Autodesk Inventor part; units mm, degrees
ref_plane "YZ Plane" through (0, 0, 0) normal (1, 0, 0) x (0, 1, 0)
ref_plane "XZ Plane" through (0, 0, 0) normal (0, 1, 0) x (-1, 0, 0)
ref_plane "XY Plane" through (0, 0, 0) normal (0, 0, 1) x (1, 0, 0)
ref_plane "작업 평면1" through (0, 0, 0) normal (0, 0, 1) x (1, 0, 0)
sketch "스케치1" plane through (0, 0, 0) normal (0, 0, 1) x (1, 0, 0)
  circle A0 centre (16.6, 17) radius 1.35
  circle A1 centre (-16.6, 17) radius 1.35
  line L0 (-49.8, -20) -> (49.8, -20)
  line L1 (49.8, -20) -> (49.8, 20)
  line L2 (49.8, 20) -> (-49.8, 20)
  line L3 (-49.8, 20) -> (-49.8, -20)
  circle A2 centre (40.6, -17) radius 1.35
  circle A3 centre (30.7755, -17) radius 1.35
  circle A4 centre (-40.6, -17) radius 1.35
  circle A5 centre (-30.7755, -17) radius 1.35
  line L4 (-49.8, 20) -> (-49.8, 14)
  line L5 (-49.8, 14) -> (49.8, 14)
  point P0 (0, 0)
  dimension "d0" = 6
extrude "돌출1" add sketch "스케치1" along normal blind 30 contours L3 L2 L1 L5
sketch "스케치2" plane through (-49.8, 20, 0) normal (0, 1, 0) x (1, 0, 0)
  line L0 (34.55, -30) -> (34.55, 0)
  line L1 (31.85, -30) -> (31.85, 0)
  line L2 (65.05, -30) -> (65.05, 0)
  line L3 (67.75, -30) -> (67.75, 0)
  line L4 (67.75, 0) -> (67.75, -6)
  line L5 (67.75, -6) -> (31.85, -6)
  line L6 (67.75, -6) -> (66.4, -6)
  line L7 (34.55, -6) -> (33.2, -6)
  line L8 (64.4, -5) -> (68.4, -5)
  line L9 (68.4, -5) -> (68.4, -7)
  line L10 (68.4, -7) -> (64.4, -7)
  line L11 (64.4, -7) -> (64.4, -5)
  line L12 (64.4, -5) -> (68.4, -7) construction
  line L13 (68.4, -5) -> (64.4, -7) construction
  line L14 (31.2, -5) -> (35.2, -5)
  line L15 (35.2, -5) -> (35.2, -7)
  line L16 (35.2, -7) -> (31.2, -7)
  line L17 (31.2, -7) -> (31.2, -5)
  line L18 (31.2, -5) -> (35.2, -7) construction
  line L19 (35.2, -5) -> (31.2, -7) construction
  point P0 (49.8, 0)
  point P1 (65.05, -6)
  dimension "d3" = 6
  dimension "d4" = 1.35
  dimension "d5" = 1.35
  dimension "d6" = 4
  dimension "d7" = 2
  dimension "d8" = 4
  dimension "d9" = 2
extrude "돌출2" cut sketch "스케치2" against normal up to surface (6 mm away)
sketch "스케치3" plane through (-49.8, 14, 0) normal (-1, 0, 0) x (0, 0, 1)
  line L0 (0, 6) -> (0, 0)
  line L1 (0, 0) -> (30, 0)
  line L2 (30, 6) -> (30, 0)
  line L3 (0, 6) -> (30, 6)
  point P0 (0, -14)
extrude "돌출3" add sketch "스케치3" along normal blind 11.7
sketch "스케치4" plane through (49.8, 14, 0) normal (1, 0, 0) x (0, 0, -1)
  line L0 (0, 0) -> (0, 6)
  line L1 (0, 6) -> (-30, 6)
  line L2 (-30, 0) -> (-30, 6)
  line L3 (0, 0) -> (-30, 0)
  point P0 (0, -14)
extrude "돌출4" add sketch "스케치4" along normal blind 11.7
sketch "스케치5" plane through (-61.5, 20, 30) normal (0, 1, 0) x (1, 0, 0)
  line L0 (42.9, 25) -> (46.9, 25)
  line L1 (46.9, 25) -> (46.9, 23)
  line L2 (46.9, 23) -> (42.9, 23)
  line L3 (42.9, 23) -> (42.9, 25)
  line L4 (80.1, 25) -> (80.1, 23)
  line L5 (80.1, 23) -> (76.1, 23)
  line L6 (76.1, 23) -> (76.1, 25)
  line L7 (76.1, 25) -> (80.1, 25)
  line L8 (0, 30) -> (123, 30)
  line L9 (0, 0) -> (0, 30)
  line L10 (0, 0) -> (123, 0)
  line L11 (123, 30) -> (123, 0)
  line L12 (0, 30) -> (3, 30)
  line L13 (3, 30) -> (3, 0)
  line L14 (123, 30) -> (120, 30)
  line L15 (120, 30) -> (120, 0)
  line L16 (0, 15) -> (123, 15)
  line L17 (3, 15) -> (3, 11)
  line L18 (3, 11) -> (123, 11)
  line L19 (3, 11) -> (3, 19)
  line L20 (3, 19) -> (9, 19)
  line L21 (9, 19) -> (9, 11)
  line L22 (9, 11) -> (3, 11)
  line L23 (120, 11) -> (120, 19)
  line L24 (120, 19) -> (114, 19)
  line L25 (114, 19) -> (114, 11)
  line L26 (114, 11) -> (120, 11)
  line L27 (3, 19) -> (9, 11)
  line L28 (3, 11) -> (9, 19)
  line L29 (114, 19) -> (120, 11)
  line L30 (114, 11) -> (120, 19)
  circle A0 centre (6, 15) radius 1.35
  circle A1 centre (117, 15) radius 1.35
  point P0 (61.5, 30)
  point P1 (120, 15)
  point P2 (9, 11)
  dimension "d16" = 3
  dimension "d17" = 3
  dimension "d18" = 4
  dimension "d19" = 8
  dimension "d20" = 6
  dimension "d21" = 6
  dimension "d24" = 2.7
  dimension "d25" = 2.7
extrude "돌출6" cut sketch "스케치5" against normal up to surface (6 mm away) contours A0 L28 L27 | L27 L16 A0 | L16 L28 A0 | A1 L16 L30 | L30 L29 A1 | A0 L16 L28 | L16 A0 L27 | L27 A0 L28 | A1 L29 L16 | L29 L16 A1 | L30 A1 L16 | L29 A1 L30
fillet "모깎기1" radius 2 4 edges at (61.5, 17, 30) (61.5, 17, 0) (-61.5, 17, 0) (-61.5, 17, 30)
properties part number "_battery_adt_2_"
Verification items for the finished model (mm, model axes). A direction names the side the tool comes from. Coordinates: 2 decimals unless noted, no trailing zeros. Loops run counter-clockwise (first coordinate to the right, second up) from the corner with the lowest first, then second, coordinate; pieces in that order, holes last. Notation, with made-up numbers: (50, 84.25) -> (104, 84.25) arc R30 ccw to (104, 115.25) -> close; hole circle Ø9 at (26, 69.25). An arc over 180 degrees is marked (long way). Answer as a JSON object with one key per item and string values. Group by question number.
Item 1: Sectioned sample at B-B on x = -55.5. Record the boundary of the cut face in (y, z), plus the area to 3 significant figures.
Item 2: Sectioned sample at A-A on y = 17. State how many separate pieces and enclosed holes the cut face has, plus the area to 3 significant figures.
Item 3: Mould release check, pull along Z, two halves, no side actions. Record for faces 3 (the flat face through (-1, 17, 0)), 4 (the flat face through (-14.6, 17, 6)), 5 (the cylindrical face through (15.605, 16.088, 2.465)): +Z half, -Z half, draft (parallel to the pull), parting line (faces both ways), or undercut.
Item 4: Tool access check on faces 1 (the flat face through (-15, 17, 7)), 2 (the flat face through (-1, 14, 15)). Record the directions out of +Z, -Z, +X, -X, +Y, -Y that give a thin tool (end or side, any length) a straight path to the whole face; none if there is none.
Item 5: Depth check by flat-ended pin: pin 1 (3 mm diameter, centred on x = 16.6, y = 17, fed in from +Z). Enter the tip coordinate at first touch or a pass-through.
Item 6: Sectioned sample at D-D on x = 16.6. Record the boundary of the cut face in (y, z), plus the area to 3 significant figures.
Item 7: Sectioned sample at C-C on z = 15. Record the boundary of the cut face in (x, y), plus the area to 3 significant figures.
Item 8: Scan lines: probe 1 along X at (y, z) = (17, 20.5); probe 2 along X at (y, z) = (18.6, 15); probe 3 along Z at (x, y) = (-17.5, 19.7). Record each from-to range of solid material in increasing order.
Evaluation:
{
 "1": {"outline": "(14, 0) -> (20, 0) -> (20, 13.65) -> (14, 13.65) -> close; (14, 16.35) -> (20, 16.35) -> (20, 30) -> (14, 30) -> close", "area": "164 mm²"},
 "2": {"separate pieces": "3", "enclosed holes": "2", "area": "3,510 mm²"},
 "3": {"face 3": "-Z half", "face 4": "undercut", "face 5": "draft"},
 "4": {"face 1": "+Y, -Y", "face 2": "+Z, -Z, +X, -X, -Y"},
 "5": {"pin 1": "stops at z = 30"},
 "6": {"outline": "(14, 0) -> (15.65, 0) -> (15.65, 5) -> (14, 5) -> close; (14, 7) -> (15.65, 7) -> (15.65, 30) -> (14, 30) -> close; (18.35, 0) -> (20, 0) -> (20, 5) -> (18.35, 5) -> close; (18.35, 7) -> (20, 7) -> (20, 30) -> (18.35, 30) -> close", "area": "92.4 mm²"},
 "7": {"outline": "(-61.5, 14) -> (-56.85, 14) -> (-56.85, 20) -> (-61.5, 20) -> close; (-54.15, 14) -> (54.15, 14) -> (54.15, 20) -> (-54.15, 20) -> close; (56.85, 14) -> (61.5, 14) -> (61.5, 20) -> (56.85, 20) -> close; hole circle Ø2.7 at (-16.6, 17); hole circle Ø2.7 at (16.6, 17)", "area": "694 mm²"},
 "8": {"probe 1": "x = -61.5 to -17.95, -15.25 to 15.25, 17.95 to 61.5", "probe 2": "x = -61.5 to -56.85, -54.15 to 54.15, 56.85 to 61.5", "probe 3": "z = 0 to 5, 7 to 30"}
}
